```python
from build123d import *

# Parameters (mm, degrees)
SKETCH1_W           = 104.775
SKETCH1_H           = 114.3
BOSS_EXTRUDE1_DEPTH = 3.175
SKETCH2_R           = 1.7526
CUT_EXTRUDE1_DEPTH  = 78.592868753
SKETCH3_R           = 2
CUT_EXTRUDE2_DEPTH  = 78.592868753
SKETCH4_R           = 1.27
CUT_EXTRUDE3_DEPTH  = 78.592868753
SKETCH5_W           = 104.775
SKETCH5_H           = 49.262233524
CUT_EXTRUDE4_DEPTH  = 15
CUT_EXTRUDE5_DEPTH  = 78.592868753


with BuildPart() as part:
    # Sketch1 → Boss-Extrude1 (new body)
    with BuildSketch(Plane.XY):
        Rectangle(SKETCH1_W, SKETCH1_H)
    extrude(amount=BOSS_EXTRUDE1_DEPTH)

    # Sketch2 → Cut-Extrude1 (cut, through all)
    with BuildSketch(Plane.XY.offset(3.175)):
        with Locations((-43.18, 15.24)):
            Circle(SKETCH2_R)
        with Locations((5.08, 15.24)):
            Circle(SKETCH2_R)
        with Locations((-40.005, -50.8762)):
            Circle(SKETCH2_R)
        with Locations((1.905, -50.8762)):
            Circle(SKETCH2_R)
    extrude(amount=-CUT_EXTRUDE1_DEPTH, mode=Mode.SUBTRACT)

    # Sketch3 → Cut-Extrude2 (cut, through all)
    with BuildSketch(Plane.XY.offset(3.175)):
        with Locations((-47.625, 22.225)):
            Circle(SKETCH3_R)
        with Locations((47.625, 22.225)):
            Circle(SKETCH3_R)
        with Locations((47.625, -28.575)):
            Circle(SKETCH3_R)
        with Locations((-47.625, -28.575)):
            Circle(SKETCH3_R)
    extrude(amount=-CUT_EXTRUDE2_DEPTH, mode=Mode.SUBTRACT)

    # Sketch4 → Cut-Extrude3 (cut, through all)
    with BuildSketch(Plane.XY.offset(3.175)):
        with Locations((18.415, -17.78)):
            Circle(SKETCH4_R)
        with Locations((38.735, -17.78)):
            Circle(SKETCH4_R)
        with Locations((38.735, -52.07)):
            Circle(SKETCH4_R)
        with Locations((18.415, -52.07)):
            Circle(SKETCH4_R)
    extrude(amount=-CUT_EXTRUDE3_DEPTH, mode=Mode.SUBTRACT)

    # Sketch5 → Cut-Extrude4 (cut)
    with BuildSketch(Plane.XY.offset(3.175)):
        with Locations((0, 57.15)):
            Rectangle(SKETCH5_W, SKETCH5_H)
    extrude(amount=-CUT_EXTRUDE4_DEPTH, mode=Mode.SUBTRACT)

    # Sketch7 → Cut-Extrude5 (cut, through all)
    with BuildSketch(Plane.XY.offset(3.175)):
        with BuildLine():
            Line((-44.45, 4.92426118), (-44.45, -14.12573882))
            ThreePointArc((-44.45, -14.12573882), (-46.0375, -15.71323882), (-47.625, -14.12573882))
            Line((-47.625, -14.12573882), (-47.625, 4.92426118))
            ThreePointArc((-47.625, 4.92426118), (-46.0375, 6.51176118), (-44.45, 4.92426118))
        make_face()
        with BuildLine():
            Line((-36.5125, 27.756383238), (26.9875, 27.756383238))
            ThreePointArc((26.9875, 27.756383238), (28.575, 26.168883238), (26.9875, 24.581383238))
            Line((26.9875, 24.581383238), (-36.5125, 24.581383238))
            ThreePointArc((-36.5125, 24.581383238), (-38.1, 26.168883238), (-36.5125, 27.756383238))
        make_face()
        with BuildLine():
            Line((28.575, 8.09926118), (28.575, -4.60073882))
            ThreePointArc((28.575, -4.60073882), (26.9875, -6.18823882), (25.4, -4.60073882))
            Line((25.4, -4.60073882), (25.4, 8.09926118))
            ThreePointArc((25.4, 8.09926118), (26.9875, 9.68676118), (28.575, 8.09926118))
        make_face()
    extrude(amount=-CUT_EXTRUDE5_DEPTH, mode=Mode.SUBTRACT)


solid = part.part
```
Verification items for the finished model (mm, model axes). A direction names the side the tool comes from. Give positions to 0.01 mm unless a question says otherwise; leave off trailing zeros. Order: outer loops, then holes, each group sorted by start corner. A loop starts at its lowest first (then second) coordinate and runs counter-clockwise, first axis right, second up. Notation, with made-up numbers: M -8.75,-27.75 L 26.25,-27.75 A21 cw 26.25,-18.75 Z; hole C 23,-21.75 d6. An arc over 180 degrees is marked long. Answer in a Markdown table with one row per item. Add a question column.
Item 1: Tool access check on faces 1 (the flat face through (-4, 24.581, 2)), 2 (the flat face through (-1, -12, 3.175)). Record the directions out of +Z, -Z, +X, -X, +Y, -Y that give a thin tool (end or side, any length) a straight path to the whole face; none if there is none.
Item 2: Section check A-A, the plane x = -3. Enter the section's corners in (y, z) (3 decimals), and give its area (3 significant figures).
Item 3: Mould release check, pull along Y, two halves, no side actions. Record for faces 3 (the cylindrical face through (18.14, -19.02, 1.61)), 4 (the flat face through (-1, -12, 0)): released by +Y, released by -Y, zero draft, split by the parting line, or undercut.
Item 4: Section check D-D, the plane x = -43.18. Enter the section's corners in (y, z) (3 decimals), and give its area (3 significant figures).
Item 5: Scan lines: probe 1 along Y at (x, z) = (2, 1.75); probe 2 along X at (y, z) = (5, 1.95) (1 decimal); probe 3 along Y at (x, z) = (22.5, 2.6). Record each from-to range of solid material in increasing order. Write a range as from..to.
Item 6: Section check B-B, the plane y = -17.78. Enter the section's corners in (x, z) (1 decimal), and give its area (3 significant figures).
Item 7: Section check C-C, the plane z = 1.5. State how many separate pieces and enclosed holes the cut face has, and give its area (3 significant figures).
Filled sheet:
| question | item | result |
|---|---|---|
| 1 | face 1 | +Z, -Z |
| 1 | face 2 | +Z, +X, -X, +Y, -Y |
| 2 | outline | M -57.15,0 L 24.581,0 L 24.581,3.175 L -57.15,3.175 Z; M 27.756,0 L 32.519,0 L 32.519,3.175 L 27.756,3.175 Z |
| 2 | area | 275 mm^2 |
| 3 | face 3 | undercut |
| 3 | face 4 | zero draft |
| 4 | outline | M -57.15,0 L 13.487,0 L 13.487,3.175 L -57.15,3.175 Z; M 16.993,0 L 32.519,0 L 32.519,3.175 L 16.993,3.175 Z |
| 4 | area | 274 mm^2 |
| 5 | probe 1 | y = -57.15..-52.63, -49.13..24.58, 27.76..32.52 |
| 5 | probe 2 | x = -52.4..-47.6, -44.5..25.4, 28.6..52.4 |
| 5 | probe 3 | y = -57.15..24.58, 27.76..32.52 |
| 6 | outline | M -52.4,0 L 17.1,0 L 17.1,3.2 L -52.4,3.2 Z; M 19.7,0 L 37.5,0 L 37.5,3.2 L 19.7,3.2 Z; M 40,0 L 52.4,0 L 52.4,3.2 L 40,3.2 Z |
| 6 | area | 317 mm^2 |
| 7 | separate pieces | 1 |
| 7 | enclosed holes | 15 |
| 7 | area | 8,960 mm^2 |
